```python
from build123d import *

# Parameters (mm, degrees)
SKETCH1_W           = 29.7
SKETCH1_H           = 11.9
BOSS_EXTRUDE1_DEPTH = 5.95
SKETCH2_R           = 1.7
CUT_EXTRUDE1_DEPTH  = 20.938279765
CUT_EXTRUDE2_DEPTH  = 0.9
SKETCH4_R           = 1.7
CUT_EXTRUDE3_DEPTH  = 20.938279765
CUT_EXTRUDE4_DEPTH  = 0.9
FILLET1_R           = 3


with BuildPart() as part:
    # Sketch1 → Boss-Extrude1 (new, symmetric)
    with BuildSketch(Plane(origin=(0, 0, 0), x_dir=(1, 0, 0), z_dir=(0, 1, 0))):
        Rectangle(SKETCH1_W, SKETCH1_H)
    extrude(amount=BOSS_EXTRUDE1_DEPTH, both=True)

    # Sketch2 → Cut-Extrude1 (cut, through all)
    with BuildSketch(Plane.XY.offset(5.95)):
        with Locations((-8.9, 0)):
            Circle(SKETCH2_R)
    cut_extrude1 = extrude(amount=-CUT_EXTRUDE1_DEPTH, mode=Mode.SUBTRACT)

    # Sketch3 → Cut-Extrude2 (cut, symmetric)
    with BuildSketch(Plane.XY):
        Polygon((-11.85, 2.95), (-11.85, 5.95), (-5.95, 5.95), (-5.95, 2.95), (-5.95, -2.95), (-11.85, -2.95), align=None)
    cut_extrude2 = extrude(amount=CUT_EXTRUDE2_DEPTH, both=True, mode=Mode.SUBTRACT)

    # Mirror1: Cut-Extrude1, Cut-Extrude2 across plane
    add(cut_extrude1.mirror(Plane(origin=(0, 0, 0), x_dir=(0, 0, 1), z_dir=(1, 0, 0))), mode=Mode.SUBTRACT)
    add(cut_extrude2.mirror(Plane(origin=(0, 0, 0), x_dir=(0, 0, 1), z_dir=(1, 0, 0))), mode=Mode.SUBTRACT)

    # Sketch4 → Cut-Extrude3 (cut, through all)
    with BuildSketch(Plane(origin=(0, 5.95, 0), x_dir=(1, 0, 0), z_dir=(0, 1, 0))):
        with Locations(Location((0, 0, 0), (0, 0, 270))):
            Circle(SKETCH4_R)
    extrude(amount=-CUT_EXTRUDE3_DEPTH, mode=Mode.SUBTRACT)

    # Sketch5 → Cut-Extrude4 (cut, symmetric)
    with BuildSketch(Plane(origin=(0, 0, 0), x_dir=(1, 0, 0), z_dir=(0, 1, 0))):
        Polygon((-2.95, 2.95), (-2.95, 5.95), (2.95, 5.95), (2.95, 2.95), (2.95, -2.95), (-2.95, -2.95), align=None)
    extrude(amount=CUT_EXTRUDE4_DEPTH, both=True, mode=Mode.SUBTRACT)

    # Fillet1
    fillet1_edges = [part.edges().sort_by_distance(p)[0] for p in [
        (-14.85, 0, -5.95),
        (14.85, 0, -5.95),
    ]]
    fillet(fillet1_edges, radius=FILLET1_R)


solid = part.part
```
Model file for the job. Use its own axes, mm. A direction names the side the tool comes from. Round coordinates to 2 decimals unless told otherwise and drop trailing zeros. Loops run counter-clockwise (first coordinate to the right, second up) from the corner with the lowest first, then second, coordinate; pieces in that order, holes last. Notation, with made-up numbers: M -15,-28.75 L 12,-28.75 A8 cw 12,-21.75 Z; hole C -37.75,65 d1. An arc over 180 degrees is marked long. Put each result on its own line as item: value. Start each with the question number.
Item 1: 3-axis set-ups, long thin cutter, end or side, ignore diameter. For faces 4 (the face through (0, -0.9, -3)), 5 (the face through (9, 3, 0.9)), 6 (the face through (-1.66, 3.46, -0.37)): which of +Z, -Z, +X, -X, +Y, -Y reach the whole face in a straight line?
Item 2: Mould opens along Z. For faces 1 (the face through (9, -2.95, 0)), 2 (the face through (7.28, 0.51, -3.39)), 3 (the face through (0, 0, 2.95)) say: released by +Z, released by -Z, zero draft, split by the parting line, or undercut.
Item 3: Cut at C-C (x = -8.9). List the corners of the cut face in (y, z), then the cut area to 4 significant figures.
Item 4: Cut at A-A (z = 0). List the corners of the cut face in (x, y).
Item 5: Drill centre lines: line 1 along X through (y, z) = (1.25, 1.5); line 2 along Y through (x, z) = (-1.5, -4.25); line 3 along Y through (x, z) = (-8.9, -2.15). Where is each one in solid material? Low to high.
Item 6: Cut at D-D (y = 3). List the corners of the cut face in (x, z).
Item 7: Drop flat-ended pins along their axis: P1, Ø3, axis at x = -8.9, y = 0, coming from the -Z side; P2, Ø0.5, axis at x = 10, z = 0, coming from the +Y side. Give the stop position or say it passes through.
Item 8: Cut at B-B (y = -3.25). List the corners of the cut face in (x, z), then the cut area to 3 significant figures.
Answer block:
1. face 4: -Z
1. face 5: +Y
1. face 6: +Y, -Y
2. face 1: undercut
2. face 2: zero draft
2. face 3: released by -Z
3. outline: M -5.95,-5.95 L -1.7,-5.95 L -1.7,-0.9 L -2.95,-0.9 L -2.95,0.9 L -1.7,0.9 L -1.7,5.95 L -5.95,5.95 Z; M 1.7,-5.95 L 5.95,-5.95 L 5.95,-0.9 L 1.7,-0.9 Z; M 1.7,0.9 L 5.95,0.9 L 5.95,5.95 L 1.7,5.95 Z
3. area: 91.25 mm2
4. outline: M -14.85,-5.95 L -1.7,-5.95 L -1.7,-0.9 L -2.95,-0.9 L -2.95,0.9 L -1.7,0.9 L -1.7,5.95 L -5.95,5.95 L -5.95,-2.95 L -11.85,-2.95 L -11.85,5.95 L -14.85,5.95 Z; M 1.7,-5.95 L 14.85,-5.95 L 14.85,5.95 L 11.85,5.95 L 11.85,-2.95 L 5.95,-2.95 L 5.95,5.95 L 1.7,5.95 L 1.7,0.9 L 2.95,0.9 L 2.95,-0.9 L 1.7,-0.9 Z
5. line 1: -14.85 to -10.05, -7.75 to -0.8, 0.8 to 7.75, 10.05 to 14.85
5. line 2: -5.95 to -0.9, 0.9 to 5.95
5. line 3: -5.95 to -1.7, 1.7 to 5.95
6. outline: M -14.85,-2.95 A3 ccw -11.85,-5.95 L 11.85,-5.95 A3 ccw 14.85,-2.95 L 14.85,5.95 L -14.85,5.95 Z; hole M -11.85,-0.9 L -5.95,-0.9 L -5.95,0.9 L -11.85,0.9 Z; hole C 0,0 d3.4; hole M 5.95,-0.9 L 11.85,-0.9 L 11.85,0.9 L 5.95,0.9 Z
7. P1: through
7. P2: y = -2.95
8. outline: M -14.85,-2.95 A3 ccw -11.85,-5.95 L 11.85,-5.95 A3 ccw 14.85,-2.95 L 14.85,5.95 L -14.85,5.95 Z; hole C 0,0 d3.4
8. area: 340 mm2
